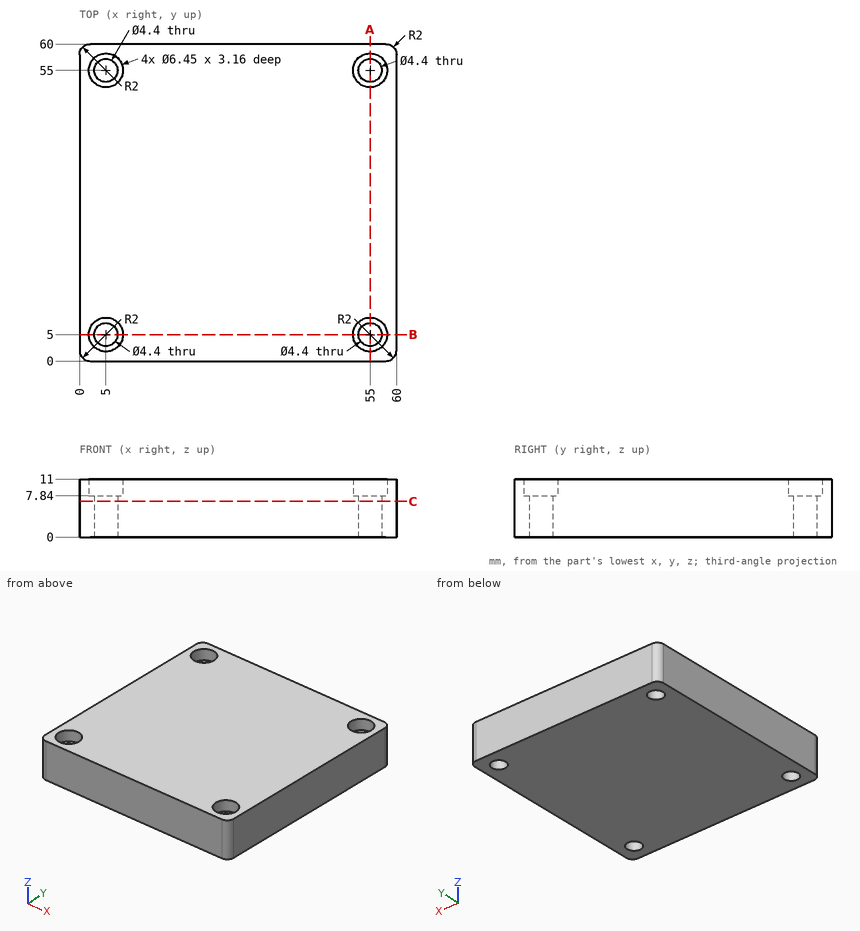
Part print with two shaded views. Sizes in mm from the minimum x, y, z corner. Round coordinates to 2 decimals unless told otherwise and drop trailing zeros. Order: outer loops, then holes, each group sorted by start corner. A loop starts at its lowest first (then second) coordinate and runs counter-clockwise, first axis right, second up. Notation, with made-up numbers: (33, 59.5) - (66, 59.5) arc R38 cw to (66, 98.5) - close; hole circle Ø9 at (35.5, 65.25). An arc over 180 degrees is marked (long way). Answer in a Markdown table with one row per item. Add a question column.
(1) Band-saw the part on C-C on z = 6.75. List the corners of the cut face in (x, y).
(2) Drop a flat-ended pin along its axis: pin 1 Ø5 at (x, y) = (55, 5) entering from +Z. Give the stop position or say it passes through.
(3) Band-saw the part on A-A on x = 55. List the corners of the cut face in (y, z) (3 decimals), and give its area (3 significant figures).
(4) Probe L1, parallel to X at y = 55, z = 10.05 (3 decimals); L2, parallel to Y at x = 5, z = 3; L3, parallel to Y at x = 6, z = 8.25. List the from-to ranges inside material, lowest first. Write a range as [from, to].
Data:
| question | item | result |
|---|---|---|
| 1 | outline | (0, 2) arc R2 ccw to (2, 0) - (58, 0) arc R2 ccw to (60, 2) - (60, 58) arc R2 ccw to (58, 60) - (2, 60) arc R2 ccw to (0, 58) - close; hole circle Ø4.4 at (5, 5); hole circle Ø4.4 at (5, 55); hole circle Ø4.4 at (55, 5); hole circle Ø4.4 at (55, 55) |
| 2 | pin 1 | stops at z = 7.84 |
| 3 | outline | (0, 0) - (2.8, 0) - (2.8, 7.84) - (1.775, 7.84) - (1.775, 11) - (0, 11) - close; (7.2, 0) - (52.8, 0) - (52.8, 7.84) - (51.775, 7.84) - (51.775, 11) - (8.225, 11) - (8.225, 7.84) - (7.2, 7.84) - close; (57.2, 0) - (60, 0) - (60, 11) - (58.225, 11) - (58.225, 7.84) - (57.2, 7.84) - close |
| 3 | area | 550 mm^2 |
| 4 | L1 | x = [0, 1.775], [8.225, 51.775], [58.225, 60] |
| 4 | L2 | y = [0, 2.8], [7.2, 52.8], [57.2, 60] |
| 4 | L3 | y = [0, 1.93], [8.07, 51.93], [58.07, 60] |
